Part model, mm, in its own coordinate system. A direction names the side the tool comes from. Give positions to 0.01 mm unless a question says otherwise; leave off trailing zeros. Order: outer loops, then holes, each group sorted by start corner. A loop starts at its lowest first (then second) coordinate and runs counter-clockwise, first axis right, second up. Notation, with made-up numbers: M 59.25,-7.5 L 79.25,-7.5 A29 ccw 79.25,23.5 Z; hole C -39,37.5 d6. An arc over 180 degrees is marked long. Return JSON: item names as keys, results as strings.
from build123d import *

# Parameters (mm, degrees)
SKETCH1_R           = 4.4
SKETCH1_R_2         = 20
BOSS_EXTRUDE1_DEPTH = 25
BOSS_EXTRUDE2_DEPTH = 5


with BuildPart() as part:
    # Sketch1 → Boss-Extrude1 (new body)
    with BuildSketch(Plane.XY):
        with BuildLine():
            Line((-50, 45), (50, 45))
            ThreePointArc((50, 45), (57.071067812, 42.071067812), (60, 35))
            Line((60, 35), (60, -35))
            ThreePointArc((60, -35), (57.071067812, -42.071067812), (50, -45))
            Line((50, -45), (-50, -45))
            ThreePointArc((-50, -45), (-57.071067812, -42.071067812), (-60, -35))
            Line((-60, -35), (-60, 35))
            ThreePointArc((-60, 35), (-57.071067812, 42.071067812), (-50, 45))
        make_face()
        with Locations((-27.5, 22.5)):
            Circle(SKETCH1_R, mode=Mode.SUBTRACT)
        with Locations((27.5, 22.5)):
            Circle(SKETCH1_R, mode=Mode.SUBTRACT)
        with Locations((-27.5, -22.5)):
            Circle(SKETCH1_R, mode=Mode.SUBTRACT)
        with Locations((27.5, -22.5)):
            Circle(SKETCH1_R, mode=Mode.SUBTRACT)
        Circle(SKETCH1_R_2, mode=Mode.SUBTRACT)
    extrude(amount=BOSS_EXTRUDE1_DEPTH)

    # Sketch2 → Boss-Extrude2 (add)
    with BuildSketch(Plane(origin=(0, 0, 0), x_dir=(-1, 0, 0), z_dir=(0, 0, -1))):
        with BuildLine():
            Line((-50.3, 44.995498987), (-50.3, -44.995498987))
            ThreePointArc((-50.3, -44.995498987), (-57.176350047, -41.964194139), (-60, -35))
            Line((-60, -35), (-60, 35))
            ThreePointArc((-60, 35), (-57.176350047, 41.964194139), (-50.3, 44.995498987))
        make_face()
        with BuildLine():
            Line((60, -35), (60, 35))
            ThreePointArc((60, 35), (57.176350047, 41.964194139), (50.3, 44.995498987))
            Line((50.3, 44.995498987), (50.3, -44.995498987))
            ThreePointArc((50.3, -44.995498987), (57.176350047, -41.964194139), (60, -35))
        make_face()
    extrude(amount=BOSS_EXTRUDE2_DEPTH)


solid = part.part
Q1. Band-saw the part on D-D (x = 0). Give the cut face in (y, z), then the cut area to 3 significant figures.
Established:
{"outline": "M -45,0 L -20,0 L -20,25 L -45,25 Z; M 20,0 L 45,0 L 45,25 L 20,25 Z", "area": "1,250 mm²"}
Q2. Band-saw the part on B-B (z = 12.25). Give the cut face in (x, y).
Established:
{"outline": "M -60,-35 A10 ccw -50,-45 L 50,-45 A10 ccw 60,-35 L 60,35 A10 ccw 50,45 L -50,45 A10 ccw -60,35 Z; hole C -27.5,-22.5 d8.8; hole C -27.5,22.5 d8.8; hole C 0,0 d40; hole C 27.5,-22.5 d8.8; hole C 27.5,22.5 d8.8"}
Q3. Pin check, flat tips, straight feed: pin 1 (4 mm diameter, centred on x = -22.5, y = 20, fed in from -Z); pin 2 (11.5 mm diameter, centred on x = 27.5, y = -22.5, fed in from +Z); pin 3 (8 mm diameter, centred on x = 27.5, y = 22.5, fed in from +Z) (3 decimals). Stop position of each tip, or through.
Established:
{"pin 1": "stops at z = 0", "pin 2": "stops at z = 25", "pin 3": "passes through"}
Q4. Band-saw the part on A-A (x = -27.5). Give the cut face in (y, z).
Established:
{"outline": "M -45,0 L -26.9,0 L -26.9,25 L -45,25 Z; M -18.1,0 L 18.1,0 L 18.1,25 L -18.1,25 Z; M 26.9,0 L 45,0 L 45,25 L 26.9,25 Z"}
Q5. Probe line 1 along X through (y, z) = (24.5, -0.25); line 2 along Y through (x, z) = (-27.5, 16.25); line 3 along Z through (x, y) = (3, 35.5). List the from-to ranges inside material, lowest first.
Established:
{"line 1": "x = -60 to -50.3, 50.3 to 60", "line 2": "y = -45 to -26.9, -18.1 to 18.1, 26.9 to 45", "line 3": "z = 0 to 25"}
Q6. Band-saw the part on C-C (y = 22.5). Give the cut face in (x, z), then the cut area to 3 significant figures.
Established:
{"outline": "M -60,-5 L -50.3,-5 L -50.3,0 L -31.9,0 L -31.9,25 L -60,25 Z; M -23.1,0 L 23.1,0 L 23.1,25 L -23.1,25 Z; M 31.9,0 L 50.3,0 L 50.3,-5 L 60,-5 L 60,25 L 31.9,25 Z", "area": "2,660 mm²"}
Q7. Two-plate mould, pull along X, no slides. Class faces 3 (the flat face through (-60, 0, 10)), 4 (the cylindrical face through (-23.436, -24.185, 12.325)), 5 (the flat face through (55, 1, -5)): +X half, -X half, draft (parallel to the pull), parting line (faces both ways), or undercut.
Established:
{"face 3": "-X half", "face 4": "undercut", "face 5": "draft"}
Q8. 3-axis set-ups, long thin cutter, end or side, ignore diameter. For faces 1 (the flat face through (1, 21, 0)), 2 (the cylindrical face through (-23.436, 20.815, 12.325)): which of +Z, -Z, +X, -X, +Y, -Y reach the whole face in a straight line?
Established:
{"face 1": "-Z, +Y, -Y", "face 2": "+Z, -Z"}
